Build history of the part. All positions in model axes, mm. Face numbers are marked on the shaded views. A direction names the side the tool comes from. Give positions to 0.01 mm unless a question says otherwise; leave off trailing zeros. Loops run counter-clockwise (first coordinate to the right, second up) from the corner with the lowest first, then second, coordinate; pieces in that order, holes last.
1) 3-axis set-ups, long thin cutter, end or side, ignore diameter. For the marked faces 4, 5 and 6: which of +Z, -Z, +X, -X, +Y, -Y reach the whole face in a straight line?
2) Two-plate mould, pull along Z, no slides. Class the marked faces 1, 2 and 3: +Z half, -Z half, draft (parallel to the pull), parting line (faces both ways), or undercut.
3) Flat gauge pins, fed straight in: P1, Ø5, axis at x = -14.5, y = 23, coming from the +Z side; P2, Ø1.5, axis at x = 14, z = 0.5, coming from the -Y side; P3, Ø5, axis at y = 4.5, z = -5, coming from the -X side. Where does each tip first touch, or does it go through?
4) Band-saw the part on C-C on x = -15. List the corners of the cut face in (y, z), then the cut area to 3 significant figures.
5) Wall check: line 1 (Z direction, x = 0, y = 5); line 2 (Y direction, x = 2.5, z = -14); line 3 (X direction, y = 5.5, z = -1.5). Give the ranges that are in metal, low to high.
6) Band-saw the part on B-B on z = 0. List the corners of the cut face in (x, y).
7) Band-saw the part on D-D on y = 11.5. List the corners of the cut face in (x, z).
8) Band-saw the part on A-A on x = 0. List the corners of the cut face in (y, z), then the cut area to 3 significant figures.
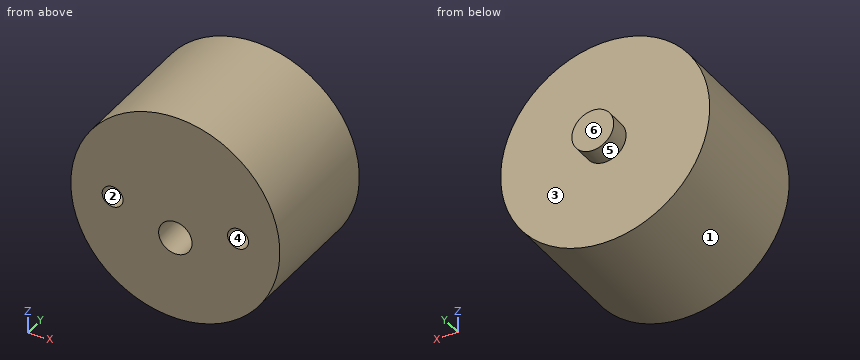
Autodesk Inventor part; units mm, degrees
ref_plane "YZ Plane" through (0, 0, 0) normal (1, 0, 0) x (0, 1, 0)
ref_plane "XZ Plane" through (0, 0, 0) normal (0, 1, 0) x (-1, 0, 0)
ref_plane "XY Plane" through (0, 0, 0) normal (0, 0, 1) x (1, 0, 0)
sketch "Sketch1" plane through (0, 0, 0) normal (0, 1, 0) x (-1, 0, 0)
  circle A0 centre (0, 0) radius 25
  dimension "d0" = 50
extrude "Extrusion1" add sketch "Sketch1" along normal blind 32
sketch "Sketch2" plane through (0, 32, 0) normal (0, 1, 0) x (1, 0, 0)
  circle A0 centre (0, 0) radius 5
  dimension "d3" = 10
extrude "Extrusion2" add sketch "Sketch2" along normal blind 5
sketch "Sketch3" plane through (0, 0, 0) normal (0, -1, 0) x (1, 0, 0)
  circle A0 centre (0, 0) radius 15
  circle A1 centre (0, 0) radius 5
  circle A2 centre (0, 0) radius 5
  point P0 (15, 0)
  point P1 (-15, 0)
  point P2 (0, -5)
  dimension "d7" = 10
  dimension "d6" = 30
hole "Hole1" at (15, 0, 0) at (-15, 0, 0) direction (0, 1, 0) diameter 5 depth 10
hole "Hole2" at (0, 0, -5) direction (0, 1, 0) diameter 8 depth 10
properties part number "stackLightBase" material "ABS Plastic"
Findings below:
1. face 4: -Y
1. face 5: +Y
1. face 6: +Z, -Z, +X, -X, +Y
2. face 1: parting line
2. face 2: undercut
2. face 3: draft
3. P1: stops at z = 21.93
3. P2: stops at y = 10
3. P3: stops at x = -24.87
4. outline: (0, -20) - (32, -20) - (32, 20) - (0, 20) - (0, 2.5) - (10, 2.5) - (10, -2.5) - (0, -2.5) - close
4. area: 1,230 mm2
5. line 1: z = -25 to -9, -1 to 25
5. line 2: y = 0 to 32
5. line 3: x = -24.95 to -17, -13 to -1.94, 1.94 to 13, 17 to 24.95
6. outline: (-25, 0) - (-17.5, 0) - (-17.5, 10) - (-12.5, 10) - (-12.5, 0) - (12.5, 0) - (12.5, 10) - (17.5, 10) - (17.5, 0) - (25, 0) - (25, 32) - (5, 32) - (5, 37) - (-5, 37) - (-5, 32) - (-25, 32) - close
7. outline: circle Ø50 at (0, 0)
8. outline: (0, -25) - (32, -25) - (32, -5) - (37, -5) - (37, 5) - (32, 5) - (32, 25) - (0, 25) - (0, -1) - (10, -1) - (10, -9) - (0, -9) - close
8. area: 1,570 mm2
